from build123d import *

# Parameters (mm, degrees)
SKETCH1_R                                           = 6
BOSS_EXTRUDE1_DEPTH                                 = 1.5
SKETCH2_R                                           = 4
SKETCH2_R_2                                         = 1.5
BOSS_EXTRUDE2_DEPTH                                 = 3
FILLET1_R                                           = 10
CSK_FOR_M4_COUNTERSUNK_FLAT_HEAD_SCREW1_D           = 4.5
CSK_FOR_M4_COUNTERSUNK_FLAT_HEAD_SCREW1_DEPTH       = 7.5
CSK_FOR_M4_COUNTERSUNK_FLAT_HEAD_SCREW1_CSINK_D     = 9.4
CSK_FOR_M4_COUNTERSUNK_FLAT_HEAD_SCREW1_CSINK_ANGLE = 90
CSK_FOR_M4_COUNTERSUNK_FLAT_HEAD_SCREW1_TIP         = 1.351936393
CUT_EXTRUDE1_DEPTH                                  = 44.802054894
FILLET2_R                                           = 10
SKETCH7_R                                           = 6
BOSS_EXTRUDE6_DEPTH                                 = 3
SKETCH10_R                                          = 1.5
BOSS_EXTRUDE7_DEPTH                                 = 3
BOSS_EXTRUDE8_DEPTH                                 = 3
FILLET3_R                                           = 1


with BuildPart() as part:
    # Sketch1 → Boss-Extrude1 (new, symmetric)
    with BuildSketch(Plane.XY):
        with BuildLine():
            Line((-25.4, -5.5), (-12.834896467, -5.5))
            ThreePointArc((-12.834896467, -5.5), (-9.445323242, -6.091982496), (-6.457063621, -7.797841329))
            ThreePointArc((-6.457063621, -7.797841329), (0, -10.124228366), (6.457063621, -7.797841329))
            ThreePointArc((6.457063621, -7.797841329), (9.445323242, -6.091982496), (12.834896467, -5.5))
            Line((12.834896467, -5.5), (25.4, -5.5))
            ThreePointArc((25.4, -5.5), (29.289087297, -3.889087297), (30.9, 0))
            ThreePointArc((30.9, 0), (0, 30.9), (-30.9, 0))
            ThreePointArc((-30.9, 0), (-29.289087297, -3.889087297), (-25.4, -5.5))
        make_face()
        Circle(SKETCH1_R, mode=Mode.SUBTRACT)
    extrude(amount=BOSS_EXTRUDE1_DEPTH, both=True)

    # Sketch2 → Boss-Extrude2 (add, through all)
    with BuildSketch(Plane.XY.offset(1.5)):
        with Locations((-26.9, 18.059623473)):
            Circle(SKETCH2_R)
        with Locations((-26.9, 18.059623473)):
            Circle(SKETCH2_R_2, mode=Mode.SUBTRACT)
    extrude(amount=-BOSS_EXTRUDE2_DEPTH)

    # Fillet1
    fillet1_edges = [part.edges().sort_by_distance(p)[0] for p in [
        (-27.493457726, 14.10389245, 0),
        (-23.463459093, 20.106618, 0),
    ]]
    fillet(fillet1_edges, radius=FILLET1_R)

    # CSK for M4 Countersunk Flat Head Screw1
    with Locations(Plane(origin=(0, 0, -1.5), x_dir=(-1, 0, 0), z_dir=(0, 0, -1))):
        with Locations((-23.4, 0), (23.4, 0)):
            CounterSinkHole(CSK_FOR_M4_COUNTERSUNK_FLAT_HEAD_SCREW1_D / 2, CSK_FOR_M4_COUNTERSUNK_FLAT_HEAD_SCREW1_CSINK_D / 2, depth=CSK_FOR_M4_COUNTERSUNK_FLAT_HEAD_SCREW1_DEPTH, counter_sink_angle=CSK_FOR_M4_COUNTERSUNK_FLAT_HEAD_SCREW1_CSINK_ANGLE)
            with Locations((0, 0, -(CSK_FOR_M4_COUNTERSUNK_FLAT_HEAD_SCREW1_DEPTH + CSK_FOR_M4_COUNTERSUNK_FLAT_HEAD_SCREW1_TIP / 2))):  # 118° drill point
                Cone(0, CSK_FOR_M4_COUNTERSUNK_FLAT_HEAD_SCREW1_D / 2, CSK_FOR_M4_COUNTERSUNK_FLAT_HEAD_SCREW1_TIP, mode=Mode.SUBTRACT)

    # Sketch6 → Cut-Extrude1 (cut, through all)
    with BuildSketch(Plane.XY.offset(1.5)):
        with BuildLine():
            Line((-17.596874723, 25.4), (17.596874723, 25.4))
            ThreePointArc((17.596874723, 25.4), (0, 30.9), (-17.596874723, 25.4))
        make_face()
    extrude(amount=-CUT_EXTRUDE1_DEPTH, mode=Mode.SUBTRACT)

    # Fillet2
    fillet2_edges = [part.edges().sort_by_distance(p)[0] for p in [
        (17.596874723, 25.4, 0),
        (-17.596874723, 25.4, 0),
    ]]
    fillet(fillet2_edges, radius=FILLET2_R)

    # Sketch7 → Boss-Extrude6 (add, through all)
    with BuildSketch(Plane(origin=(0, 0, -1.5), x_dir=(-1, 0, 0), z_dir=(0, 0, -1))):
        with BuildLine():
            Line((-14.129755837, 25.4), (-7.129755837, 25.4))
            ThreePointArc((-7.129755837, 25.4), (-19.515300955, 27.292035274), (-30.771089101, 32.795557652))
            ThreePointArc((-30.771089101, 32.795557652), (-43.404263963, 30.368503031), (-40.705792002, 17.790508346))
            ThreePointArc((-40.705792002, 17.790508346), (-33.513792252, 10.156964901), (-30.9, 0))
            ThreePointArc((-30.9, 0), (-28.287130475, 12.435764935), (-20.890404562, 22.768421053))
            ThreePointArc((-20.890404562, 22.768421053), (-17.757137087, 24.718911163), (-14.129755837, 25.4))
        make_face()
        with Locations((-35.9, 25.4)):
            Circle(SKETCH7_R, mode=Mode.SUBTRACT)
    extrude(amount=-BOSS_EXTRUDE6_DEPTH)

    # Sketch10 → Boss-Extrude7 (add, through all)
    with BuildSketch(Plane(origin=(0, 0, -1.5), x_dir=(-1, 0, 0), z_dir=(0, 0, -1))):
        with BuildLine():
            Line((-34.78083152, -5.5), (-25.4, -5.5))
            ThreePointArc((-25.4, -5.5), (-29.289087297, -3.889087297), (-30.9, 0))
            ThreePointArc((-30.9, 0), (-31.563922472, 5.243945221), (-33.513792252, 10.156964901))
            ThreePointArc((-33.513792252, 10.156964901), (-33.13038334, 5.551807562), (-36.308268134, 2.196882117))
            ThreePointArc((-36.308268134, 2.196882117), (-38.704320303, -2.278611434), (-34.78083152, -5.5))
        make_face()
        with Locations((-34.78083152, -1.5)):
            Circle(SKETCH10_R, mode=Mode.SUBTRACT)
    extrude(amount=-BOSS_EXTRUDE7_DEPTH)

    # Sketch12 → Boss-Extrude8 (add, through all)
    with BuildSketch(Plane(origin=(0, 0, -1.5), x_dir=(-1, 0, 0), z_dir=(0, 0, -1))):
        with BuildLine():
            ThreePointArc((7.813736863, 28.9), (6.788610597, 26.425126266), (4.313736863, 25.4))
            Line((4.313736863, 25.4), (14.313736863, 25.4))
            ThreePointArc((14.313736863, 25.4), (11.838863129, 26.425126266), (10.813736863, 28.9))
            Line((10.813736863, 28.9), (7.813736863, 28.9))
        make_face()
        with BuildLine():
            ThreePointArc((4.313736863, 25.4), (1.838863129, 26.425126266), (0.813736863, 28.9))
            Line((0.813736863, 28.9), (-2.186263137, 28.9))
            ThreePointArc((-2.186263137, 28.9), (-3.211389403, 26.425126266), (-5.686263137, 25.4))
            Line((-5.686263137, 25.4), (4.313736863, 25.4))
        make_face()
    extrude(amount=-BOSS_EXTRUDE8_DEPTH)

    # Fillet3
    fillet3_edges = [part.edges().sort_by_distance(p)[0] for p in [
        (-10.813736863, 28.9, 0),
        (-7.813736863, 28.9, 0),
        (2.186263137, 28.9, 0),
        (-0.813736863, 28.9, 0),
    ]]
    fillet(fillet3_edges, radius=FILLET3_R)


solid = part.part
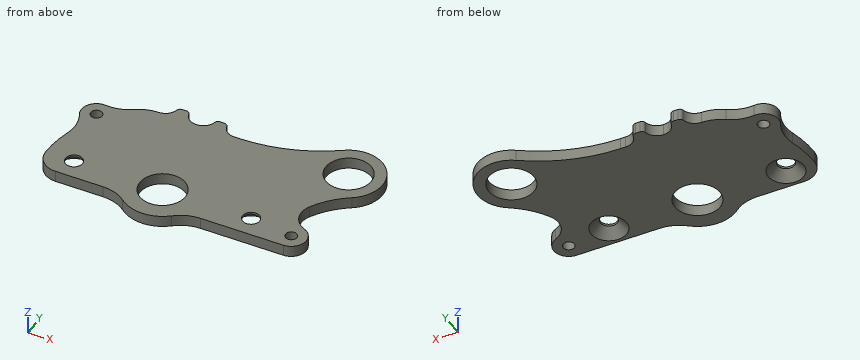
Read the model definition and answer for the solid it produces. Units are mm, in the model's axes. Give positions to 0.01 mm unless a question says otherwise; leave off trailing zeros. Write each loop counter-clockwise with the first axis right and the second up, starting at its lowest first coordinate (ties: lowest second). Pieces come first, ordered by that corner, then holes. Notation, with made-up numbers: M 2,78 L 16,78 A12 cw 16,96 Z; hole C 75.25,6.5 d6. An arc over 180 degrees is marked long. One line per item, written item: value. Start each with the question number.
(1) Find section B-B (z = 0). Give the number of separate pieces and of enclosed holes in the cut face, plus the area to 3 significant figures.
(2) Flat-ended cylindrical pins translate along their axes: pin 1 Ø1.2 at (x, z) = (6.5, 0.5) entering from +Y; pin 2 Ø14 at (x, y) = (35.9, 25.4) entering from +Z; pin 3 Ø0.6 at (x, z) = (-9.5, 0.5) entering from +Y. Find the tip coordinate at first contact, or state that the pin passes through.
(3) Find the intervals of material crossed by line 1 (X direction, y = 28.5, z = -0.7); line 2 (Y direction, x = 0, z = 0.4); line 3 (Y direction, x = -24.5, z = -1.3), in increasing order.
(4) Find section A-A (x = 23.4). Determine the outline of the cut face in (y, z).
(5) Find section C-C (x = 12). Determine the outline of the cut face in (y, z).
Results below:
1. separate pieces: 1
1. enclosed holes: 6
1. area: 2,010 mm^2
2. pin 1: stops at y = 25.4
2. pin 2: stops at z = 1.5
2. pin 3: stops at y = 28.9
3. line 1: x = -10.73 to -7.9, -0.73 to 2.1, 22.86 to 30.76, 41.04 to 44.35
3. line 2: y = -10.12 to -6, 6 to 28.9
3. line 3: y = -5.5 to -4.36, 4.36 to 22.04
4. outline: M -5.5,-1.5 L -4.7,-1.5 L -2.25,0.95 L -2.25,1.5 L -5.5,1.5 Z; M 2.25,0.95 L 4.7,-1.5 L 28.72,-1.5 L 28.72,1.5 L 2.25,1.5 Z
5. outline: M -5.53,-1.5 L 25.69,-1.5 L 25.69,1.5 L -5.53,1.5 Z
